Geometry: final body of the model. Coordinates: model frame, mm. A direction names the side the tool comes from. Give positions to 0.01 mm unless a question says otherwise; leave off trailing zeros. Write each loop counter-clockwise with the first axis right and the second up, starting at its lowest first coordinate (ties: lowest second). Pieces come first, ordered by that corner, then holes.
Q1. Pin query (flat end, axial travel): pin 1 Ø1.7 at (x, y) = (0, -7) entering from -Z; pin 2 Ø1.5 at (x, z) = (-0.5, 8) entering from +Y; pin 3 Ø1.7 at (x, y) = (7.85, -7.85) entering from +Z; pin 4 Ø2.5 at (x, z) = (5.08, 20.02) entering from -Y. Return the tip coordinate at first contact, or that it passes through.
Q2. Line query: line 1 (Z direction, x = 8.5, y = 2); line 2 (X direction, y = -18, z = 31); line 3 (Y direction, x = 4.5, z = 4). Output: solid intervals per line, ascending.
Q3. Mould query, pull axis X, two halves, no side actions, for faces 4 (the cylindrical face through (7.71, -6.81, 47.74)), 5 (the cylindrical face through (-5, -6, 2)), 6 (the flat face through (5, -23, 25)), 7 (the cylindrical face through (9.02, 4.54, 2.46)). Classes: +X half, -X half, draft (parallel to the pull), parting line (faces both ways), or undercut.
Q4. Section C-C (z = 47.5). Return the cut outline in (x, y), plus the area to 3 significant figures.
Q5. Reachability of faces 1 (the flat face through (-5, -17, 25)), 2 (the cylindrical face through (5, 3.9, 2.5)), 3 (the cylindrical face through (-8.9, 0, 47.7)) from +Z, -Z, +X, -X, +Y, -Y: full face, straight path, thin tool, end or side. Return the list, or none.
Q6. Section D-D (x = -2.25). Return the cut outline in (y, z).
Q7. Section B-B (y = -16). Return the cut outline in (x, z), plus the area to 3 significant figures.
Q8. Section A-A (z = 25.1). Return the cut outline in (x, y).
from build123d import *

# Parameters (mm, degrees)
BOSS_EXTRUDE1_DEPTH = 50.2
CUT_EXTRUDE2_DEPTH  = 44.2
SKETCH3_W           = 20.2
SKETCH3_H           = 10.1
BOSS_EXTRUDE2_DEPTH = 5
SKETCH4_R           = 1.05
CUT_EXTRUDE3_DEPTH  = 11
SKETCH5_R           = 4
SKETCH5_R_2         = 7.5
CUT_EXTRUDE4_DEPTH  = 11
SKETCH6_R           = 4
BOSS_EXTRUDE3_DEPTH = 5
SKETCH7_R           = 4
SKETCH7_R_2         = 1.05
CUT_EXTRUDE5_DEPTH  = 16
SKETCH8_R           = 7.5
CUT_EXTRUDE6_DEPTH  = 11
SKETCH9_R           = 4
BOSS_EXTRUDE4_DEPTH = 5
SKETCH11_W          = 20.2
SKETCH11_H          = 50.2
BOSS_EXTRUDE5_DEPTH = 3
SKETCH12_R          = 3
SKETCH12_R_2        = 1.55
CUT_EXTRUDE8_DEPTH  = 23


with BuildPart() as part:
    # Sketch1 → Boss-Extrude1 (new body)
    with BuildSketch(Plane.XY):
        with BuildLine():
            Line((-10.1, 0), (-10.1, -20))
            Line((-10.1, -20), (10.1, -20))
            Line((10.1, -20), (10.1, 0))
            ThreePointArc((10.1, 0), (0, 10.1), (-10.1, 0))
        make_face()
    extrude(amount=BOSS_EXTRUDE1_DEPTH)

    # Sketch2 → Cut-Extrude2 (cut)
    with BuildSketch(Plane.ZY.offset(10.1)):
        Polygon((5, -10), (5, -17), (45.2, -17), (45.2, -10), (45.2, 11.866817026), (5, 11.866817026), align=None)
    extrude(amount=-CUT_EXTRUDE2_DEPTH, mode=Mode.SUBTRACT)

    # Sketch3 → Boss-Extrude2 (add)
    with BuildSketch(Plane.XY.offset(50.2)):
        with Locations((0, 5.05)):
            Rectangle(SKETCH3_W, SKETCH3_H)
    extrude(amount=-BOSS_EXTRUDE2_DEPTH)

    # Sketch4 → Cut-Extrude3 (cut, symmetric)
    with BuildSketch(Plane.XY.offset(50.2)):
        with Locations((-7.85, 7.85)):
            Circle(SKETCH4_R)
        with Locations((7.85, 7.85)):
            Circle(SKETCH4_R)
        with Locations((-7.85, -7.85)):
            Circle(SKETCH4_R)
        with Locations((7.85, -7.85)):
            Circle(SKETCH4_R)
        with Locations((0, 7.85)):
            Circle(SKETCH4_R)
        with Locations((0, -7.85)):
            Circle(SKETCH4_R)
        with Locations((-7.85, 0)):
            Circle(SKETCH4_R)
        with Locations((7.85, 0)):
            Circle(SKETCH4_R)
    extrude(amount=CUT_EXTRUDE3_DEPTH, both=True, mode=Mode.SUBTRACT)

    # Sketch5 → Cut-Extrude4 (cut, symmetric)
    with BuildSketch(Plane.XY.offset(50.2)):
        Circle(SKETCH5_R)
        with Locations((0, 12.82)):
            Circle(SKETCH5_R_2)
    extrude(amount=CUT_EXTRUDE4_DEPTH, both=True, mode=Mode.SUBTRACT)

    # Sketch6 → Boss-Extrude3 (add)
    with BuildSketch(Plane.XY.offset(50.2)):
        Circle(SKETCH6_R)
    extrude(amount=-BOSS_EXTRUDE3_DEPTH)

    # Sketch7 → Cut-Extrude5 (cut, symmetric)
    with BuildSketch(Plane(origin=(0, 0, 0), x_dir=(-1, 0, 0), z_dir=(0, 0, -1))):
        with Locations(Location((0, 0, 0), (0, 0, 90))):
            Circle(SKETCH7_R)
        with Locations(Location((0, 7, 0), (0, 0, 90))):
            Circle(SKETCH7_R_2)
        with Locations(Location((-4.949747468, 4.949747468, 0), (0, 0, 90))):
            Circle(SKETCH7_R_2)
        with Locations(Location((-7, 0, 0), (0, 0, 90))):
            Circle(SKETCH7_R_2)
        with Locations(Location((-4.949747468, -4.949747468, 0), (0, 0, 90))):
            Circle(SKETCH7_R_2)
        with Locations(Location((0, -7, 0), (0, 0, 90))):
            Circle(SKETCH7_R_2)
        with Locations(Location((4.949747468, -4.949747468, 0), (0, 0, 90))):
            Circle(SKETCH7_R_2)
        with Locations(Location((7, 0, 0), (0, 0, 90))):
            Circle(SKETCH7_R_2)
        with Locations(Location((4.949747468, 4.949747468, 0), (0, 0, 90))):
            Circle(SKETCH7_R_2)
    extrude(amount=CUT_EXTRUDE5_DEPTH, both=True, mode=Mode.SUBTRACT)

    # Sketch8 → Cut-Extrude6 (cut, symmetric)
    with BuildSketch(Plane(origin=(0, 0, 0), x_dir=(-1, 0, 0), z_dir=(0, 0, -1))):
        with Locations((0, 12.82)):
            Circle(SKETCH8_R)
    extrude(amount=CUT_EXTRUDE6_DEPTH, both=True, mode=Mode.SUBTRACT)

    # Sketch9 → Boss-Extrude4 (add)
    with BuildSketch(Plane(origin=(0, 0, 0), x_dir=(-1, 0, 0), z_dir=(0, 0, -1))):
        Circle(SKETCH9_R)
    extrude(amount=-BOSS_EXTRUDE4_DEPTH)

    # Sketch11 → Boss-Extrude5 (add)
    with BuildSketch(Plane(origin=(0, -20, 0), x_dir=(-1, 0, 0), z_dir=(0, -1, 0))):
        with Locations((0, -25.1)):
            Rectangle(SKETCH11_W, SKETCH11_H)
    extrude(amount=BOSS_EXTRUDE5_DEPTH)

    # Sketch12 → Cut-Extrude8 (cut)
    with BuildSketch(Plane(origin=(0, -17, 0), x_dir=(1, 0, 0), z_dir=(0, 1, 0))):
        with Locations(Location((0, -25.1, 0), (0, 0, 270))):
            Circle(SKETCH12_R)
        with Locations(Location((-5.084097757, -20.015902243, 0), (0, 0, 270))):
            Circle(SKETCH12_R_2)
        with Locations(Location((5.084097757, -20.015902243, 0), (0, 0, 270))):
            Circle(SKETCH12_R_2)
        with Locations(Location((5.084097757, -30.184097757, 0), (0, 0, 270))):
            Circle(SKETCH12_R_2)
        with Locations(Location((-5.084097757, -30.184097757, 0), (0, 0, 270))):
            Circle(SKETCH12_R_2)
    extrude(amount=-CUT_EXTRUDE8_DEPTH, mode=Mode.SUBTRACT)


solid = part.part
Computed:
1. pin 1: stops at z = 45.2
1. pin 2: stops at y = -17
1. pin 3: stops at z = 5
1. pin 4: passes through
2. line 1: z = 0 to 5, 45.2 to 50.2
2. line 2: x = -10.1 to -6.4, -3.77 to 3.77, 6.4 to 10.1
2. line 3: y = -23 to -5.9, -4 to 4, 5.9 to 6.82
3. face 4: undercut
3. face 5: undercut
3. face 6: draft
3. face 7: +X half
4. outline: (-10.1, -23) - (10.1, -23) - (10.1, 10.1) - (6.99, 10.1) arc R7.5 cw to (-6.99, 10.1) - (-10.1, 10.1) - close; hole circle Ø2.1 at (-7.85, -7.85); hole circle Ø2.1 at (-7.85, 0); hole circle Ø2.1 at (-7.85, 7.85); hole circle Ø2.1 at (0, -7.85); hole circle Ø2.1 at (7.85, -7.85); hole circle Ø2.1 at (7.85, 0); hole circle Ø2.1 at (7.85, 7.85)
4. area: 596 mm2
5. face 1: +X, -X, +Y
5. face 2: -Z
5. face 3: +Z
6. outline: (-23, 0) - (5.67, 0) - (5.67, 5) - (-17, 5) - (-17, 23.12) - (-23, 23.12) - close; (-23, 27.08) - (-17, 27.08) - (-17, 45.2) - (5.67, 45.2) - (5.67, 50.2) - (-23, 50.2) - close
7. outline: (-10.1, 0) - (10.1, 0) - (10.1, 5) - (-10.1, 5) - close; (-10.1, 45.2) - (10.1, 45.2) - (10.1, 50.2) - (-10.1, 50.2) - close
7. area: 202 mm2
8. outline: (-10.1, -23) - (-3, -23) - (-3, -17) - (-10.1, -17) - close; (3, -23) - (10.1, -23) - (10.1, -17) - (3, -17) - close
